Input: part model. Units: mm. Frame: model coordinates. A direction names the side the tool comes from. Coordinates: 2 decimals unless noted, no trailing zeros. Write each loop counter-clockwise with the first axis right and the second up, starting at its lowest first coordinate (ties: lowest second). Pieces come first, ordered by that corner, then holes. Notation, with made-up numbers: M 44.5,46.25 L 50.5,46.25 A29 cw 50.5,79.25 Z; hole C 86.25,21 d4. An arc over 180 degrees is marked long. Use one line per item in the form item = value.
from build123d import *

# Parameters (mm, degrees)
SKETCH1_W                  = 107.95
SKETCH1_H                  = 222.25
BOSS_EXTRUDE1_DEPTH        = 3.175
SKETCH3_W                  = 17.3736
SKETCH3_H                  = 30.5054
SKETCH3_W_2                = 7.8994
SKETCH3_H_2                = 2.8194
SKETCH3_W_3                = 5.588
SKETCH3_H_3                = 32.2834
SKETCH3_W_4                = 6.0198
SKETCH3_H_4                = 2.6162
BOSS_EXTRUDE2_DEPTH        = 3.175
F_4_0_209_DIAMETER_HOLE1_D = 5.3086
SKETCH7_W                  = 31.75
SKETCH7_H                  = 40.64
BOSS_EXTRUDE3_DEPTH        = 3.175


with BuildPart() as part:
    # Sketch1 → Boss-Extrude1 (new body)
    with BuildSketch(Plane(origin=(0, 0, 0), x_dir=(1, 0, 0), z_dir=(0, 1, 0))):
        with Locations((53.975, 111.125)):
            Rectangle(SKETCH1_W, SKETCH1_H)
    extrude(amount=BOSS_EXTRUDE1_DEPTH)

    # Sketch3 → Boss-Extrude2 (add)
    with BuildSketch(Plane(origin=(0, 3.175, 0), x_dir=(1, 0, 0), z_dir=(0, 1, 0))):
        with Locations((2.3368, 187.3377)):
            Rectangle(SKETCH3_W, SKETCH3_H)
        with Locations((19.1897, 149.7203)):
            Rectangle(SKETCH3_W_2, SKETCH3_H_2)
        with Locations((19.1897, 74.7903)):
            Rectangle(SKETCH3_W_2, SKETCH3_H_2)
        with Locations((19.177, 38.2397)):
            Rectangle(SKETCH3_W_3, SKETCH3_H_3)
        with Locations((43.2943, 182.7657)):
            Rectangle(SKETCH3_W_4, SKETCH3_H_4)
        with Locations((43.2943, 170.0657)):
            Rectangle(SKETCH3_W_4, SKETCH3_H_4)
    extrude(amount=BOSS_EXTRUDE2_DEPTH)

    # #4 (0.209) Diameter Hole1 (through all)
    with Locations(Plane(origin=(0, 3.175, 0), x_dir=(1, 0, 0), z_dir=(0, 1, 0))):
        with Locations((101.6, 215.9), (101.6, 6.35), (6.35, 6.35), (6.35, 215.9), (6.35, 107.95), (101.6, 107.95)):
            Hole(F_4_0_209_DIAMETER_HOLE1_D / 2)

    # Sketch7 → Boss-Extrude3 (add)
    with BuildSketch(Plane(origin=(0, 6.35, 0), x_dir=(1, 0, 0), z_dir=(0, 1, 0))):
        with Locations((12.065, 38.2397)):
            Rectangle(SKETCH7_W, SKETCH7_H)
    extrude(amount=BOSS_EXTRUDE3_DEPTH)


solid = part.part
(1) Section query C-C on x = 101.6. Return the cut outline in (y, z) (3 decimals), plus the area to 3 significant figures.
Computed:
outline = M 0,-222.25 L 3.175,-222.25 L 3.175,-218.554 L 0,-218.554 Z; M 0,-213.246 L 3.175,-213.246 L 3.175,-110.604 L 0,-110.604 Z; M 0,-105.296 L 3.175,-105.296 L 3.175,-9.004 L 0,-9.004 Z; M 0,-3.696 L 3.175,-3.696 L 3.175,0 L 0,0 Z
area = 655 mm^2
(2) Line query: probe 1 along Z at (x, y) = (101.6, 1.85); probe 2 along X at (y, z) = (1.2, -215.9); probe 3 along Y at (x, z) = (7, -48) (3 decimals). Output: solid intervals per line, ascending.
Computed:
probe_1 = -222.25 to -218.55, -213.25 to -110.6, -105.3 to -9, -3.7 to 0
probe_2 = 0 to 3.7, 9 to 98.95, 104.25 to 107.95
probe_3 = 0 to 3.175, 6.35 to 9.525
(3) First-contact query: pin 1 Ø2.5 at (y, z) = (5, -186) entering from +X; pin 2 Ø1.4 at (y, z) = (5.5, -149.5) entering from -X; pin 3 Ø2 at (x, z) = (83.5, -119) entering from +Y (3 decimals). Flat tips, straight axial feed; report the tip coordinate or a pass-through.
Computed:
pin_1 = 11.02
pin_2 = 15.24
pin_3 = 3.175
(4) Pull-direction query (X, two-part tool) for faces 4 (the flat face through (12, 6.35, -39)), 5 (the cylindrical face through (103.56, 1.57, -109.74)), 6 (the cylindrical face through (4.923, 1.565, -218.138)); classes: pulls with the +X half, pulls with the -X half, needs draft (parallel to the pull), parting line crosses it, or undercut.
Computed:
face_4 = needs draft
face_5 = undercut
face_6 = undercut
(5) Section query D-D on y = 8. Return the cut outline in (x, z), plus the area to 3 significant figures.
Computed:
outline = M -3.81,-58.56 L 27.94,-58.56 L 27.94,-17.92 L -3.81,-17.92 Z
area = 1,290 mm^2
(6) Set-up query: faces 1 (the cylindrical face through (4.923, 1.565, -110.188)), 2 (the flat face through (2, 6.35, -188)), 3 (the flat face through (-3, 3.175, -188)). Return all of +Z, -Z, +X, -X, +Y, -Y with unobstructed straight access to the full face (end or side cutting, diameter ignored); none if empty.
Computed:
face_1 = +Y, -Y
face_2 = -Z, +X, -X, +Y
face_3 = +Z, -Z, -X, -Y
(7) Section query A-A on z = -215.9. Return the cut outline in (x, y) (3 decimals).
Computed:
outline = M 0,0 L 3.696,0 L 3.696,3.175 L 0,3.175 Z; M 9.004,0 L 98.946,0 L 98.946,3.175 L 9.004,3.175 Z; M 104.254,0 L 107.95,0 L 107.95,3.175 L 104.254,3.175 Z
(8) Section query B-B on x = 6.35. Return the cut outline in (y, z) (3 decimals), plus the area to 3 significant figures.
Computed:
outline = M 0,-222.25 L 3.175,-222.25 L 3.175,-218.554 L 0,-218.554 Z; M 0,-213.246 L 3.175,-213.246 L 3.175,-202.59 L 6.35,-202.59 L 6.35,-172.085 L 3.175,-172.085 L 3.175,-110.604 L 0,-110.604 Z; M 0,-105.296 L 3.175,-105.296 L 3.175,-9.004 L 0,-9.004 Z; M 0,-3.696 L 3.175,-3.696 L 3.175,0 L 0,0 Z; M 6.35,-58.56 L 9.525,-58.56 L 9.525,-17.92 L 6.35,-17.92 Z
area = 881 mm^2
